from build123d import *


with BuildPart() as part:
    # Sketch1 → Revolve1 (revolve)
    with BuildSketch(Plane.XY):
        Polygon((-8, 17.5), (-8, 15), (-7.188, 14.188), (-0.812, 14.188), (0, 15), (0, 15.8), (-1.5, 15.8), (-3.2, 17.5), align=None)
    revolve(axis=Axis((50, 0, 0), (-1, 0, 0)))

    # Sketch2 → Cut-Revolve1 (revolve, cut)
    with BuildSketch(Plane.XY):
        Polygon((-8, 17.3), (-7.8, 17.5), (0, 17.5), (0, 20), (-8, 20), align=None)
    revolve(axis=Axis((50, 0, 0), (-1, 0, 0)), mode=Mode.SUBTRACT)


solid = part.part
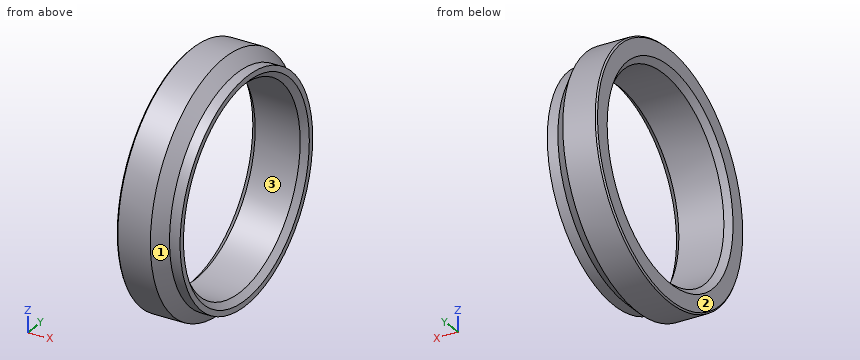
Verification items for the finished model (mm, model axes). Face numbers are marked on the shaded views. Give positions to 0.01 mm unless a question says otherwise; leave off trailing zeros. Loops run counter-clockwise (first coordinate to the right, second up) from the corner with the lowest first, then second, coordinate; pieces in that order, holes last.
1. Material ranges on probe 1 along Y at (x, z) = (-4, 0); probe 2 along Z at (x, y) = (-6, 0.5); probe 3 along Y at (x, z) = (-0.75, 6), recorded low to high.
Derived:
probe 1: y = -17.5 to -14.19, 14.19 to 17.5
probe 2: z = -17.49 to -14.18, 14.18 to 17.49
probe 3: y = -14.62 to -12.93, 12.93 to 14.62
2. Cross-section at A-A on y = 0. Record the cut outline in (x, z), and give its area (3 significant figures).
Derived:
outline: (-8, -17.3) - (-7.8, -17.5) - (-3.2, -17.5) - (-1.5, -15.8) - (0, -15.8) - (0, -15) - (-0.81, -14.19) - (-7.19, -14.19) - (-8, -15) - close; (-8, 15) - (-7.19, 14.19) - (-0.81, 14.19) - (0, 15) - (0, 15.8) - (-1.5, 15.8) - (-3.2, 17.5) - (-7.8, 17.5) - (-8, 17.3) - close
area: 43.6 mm2
3. Release check for a two-part mould opening along Y. For the marked faces 1, 2 and 3 record: +Y half, -Y half, draft (parallel to the pull), parting line (faces both ways), or undercut.
Derived:
face 1: parting line
face 2: draft
face 3: undercut
4. Go/stop test with flat-tipped pins: P1, Ø2, axis at y = 11.5, z = -5, coming from the -X side; P2, Ø1.5, axis at x = -7, y = 6.5, coming from the -Z side; P3, Ø1.5, axis at x = -2, z = -10.5, coming from the +Y side. Record where each tip stops, or that it passes through.
Derived:
P1: passes through
P2: stops at z = -16.53
P3: stops at y = 13.59
5. Cross-section at C-C on x = -5. Record the cut outline in (y, z).
Derived:
outline: circle Ø35 at (0, 0); hole circle Ø28.38 at (0, 0)
